Geometry check sheet. Reference: the model listing, model coordinates, mm. A direction names the side the tool comes from. Coordinates: 2 decimals unless noted, no trailing zeros. Write each loop counter-clockwise with the first axis right and the second up, starting at its lowest first coordinate (ties: lowest second). Pieces come first, ordered by that corner, then holes.
from build123d import *

# Parameters (mm, degrees)
SKETCH_W        = 100.5
SKETCH_H        = 50
SKETCH_R        = 1.7
SKETCH_W_2      = 30
SKETCH_H_2      = 40
SKETCH_W_3      = 13
PAD_DEPTH       = 8
SKETCH001_W     = 86.5
SKETCH001_H     = 44
POCKET_DEPTH    = 3
SKETCH002_W     = 96.5
SKETCH002_H     = 2
POCKET001_DEPTH = 4
POCKET003_DEPTH = 5
SKETCH005_R     = 1.7
POCKET004_DEPTH = 3.001
POCKET005_DEPTH = 3
FILLET_R        = 3
FILLET001_R     = 3
FILLET002_R     = 3
FILLET003_R     = 3
SKETCH007_W     = 4
SKETCH007_H     = 35
POCKET006_DEPTH = 3
SKETCH008_R     = 2
POCKET007_DEPTH = 5.001
CHAMFER_SIZE    = 1.5
CHAMFER001_SIZE = 1.5
CHAMFER002_SIZE = 1.5
CHAMFER003_SIZE = 1.5


with BuildPart() as part:
    # Sketch → Pad (new body)
    with BuildSketch(Plane.XY):
        Rectangle(SKETCH_W, SKETCH_H)
        with Locations((-6, 0)):
            Circle(SKETCH_R, mode=Mode.SUBTRACT)
        with Locations((19, 0)):
            Circle(SKETCH_R, mode=Mode.SUBTRACT)
        with Locations((-28.25, 0)):
            Rectangle(SKETCH_W_2, SKETCH_H_2, mode=Mode.SUBTRACT)
        with Locations((36.75, 0)):
            Rectangle(SKETCH_W_3, SKETCH_H_2, mode=Mode.SUBTRACT)
    extrude(amount=PAD_DEPTH)

    # Sketch001 → Pocket (cut)
    with BuildSketch(Plane.XY.offset(8)):
        Rectangle(SKETCH001_W, SKETCH001_H)
    extrude(amount=-POCKET_DEPTH, mode=Mode.SUBTRACT)

    # Sketch002 → Pocket001 (cut)
    with BuildSketch(Plane.XY.offset(8)):
        with Locations((0, 10.5)):
            Rectangle(SKETCH002_W, SKETCH002_H)
        with Locations((0, -4.5)):
            Rectangle(SKETCH002_W, SKETCH002_H)
    extrude(amount=-POCKET001_DEPTH, mode=Mode.SUBTRACT)

    # Sketch004 → Pocket003 (cut)
    with BuildSketch(Plane.XY.offset(8)):
        Polygon((-50.25, 25), (50.25, 25), (50.25, 17), (43.25, 17), (43.25, 22), (-43.25, 22), (-43.25, 17), (-50.25, 17), align=None)
        Polygon((50.25, -17), (50.25, -25), (-50.25, -25), (-50.25, -17), (-43.25, -17), (-43.25, -22), (43.25, -22), (43.25, -17), align=None)
    extrude(amount=-POCKET003_DEPTH, mode=Mode.SUBTRACT)

    # Sketch005 → Pocket004 (cut, through all)
    with BuildSketch(Plane.XY.offset(3)):
        with Locations((-47, 21)):
            Circle(SKETCH005_R)
        with Locations((47, 21)):
            Circle(SKETCH005_R)
        with Locations((47, -21)):
            Circle(SKETCH005_R)
        with Locations((-47, -21)):
            Circle(SKETCH005_R)
    extrude(amount=-POCKET004_DEPTH, mode=Mode.SUBTRACT)

    # Sketch006 → Pocket005 (cut)
    with BuildSketch(Plane.XY.offset(5)):
        Polygon((-7.587713, 2.75), (-9.175426, 0), (-7.587713, -2.75), (-4.412287, -2.75), (-2.824574, 0), (-4.412287, 2.75), align=None)
        Polygon((17.412287, 2.75), (15.824574, 0), (17.412287, -2.75), (20.587713, -2.75), (22.175426, 0), (20.587713, 2.75), align=None)
    extrude(amount=-POCKET005_DEPTH, mode=Mode.SUBTRACT)

    # Fillet
    fillet_edges = [part.edges().sort_by_distance(p)[0] for p in [
        (-50.25, -25, 1.5),
    ]]
    fillet(fillet_edges, radius=FILLET_R)

    # Fillet001
    fillet001_edges = [part.edges().sort_by_distance(p)[0] for p in [
        (-50.25, 25, 1.5),
    ]]
    fillet(fillet001_edges, radius=FILLET001_R)

    # Fillet002
    fillet002_edges = [part.edges().sort_by_distance(p)[0] for p in [
        (50.25, -25, 1.5),
    ]]
    fillet(fillet002_edges, radius=FILLET002_R)

    # Fillet003
    fillet003_edges = [part.edges().sort_by_distance(p)[0] for p in [
        (50.25, 25, 1.5),
    ]]
    fillet(fillet003_edges, radius=FILLET003_R)

    # Sketch007 → Pocket006 (cut)
    with BuildSketch(Plane.XY.offset(5)):
        with Locations((2, 0)):
            Rectangle(SKETCH007_W, SKETCH007_H)
    extrude(amount=-POCKET006_DEPTH, mode=Mode.SUBTRACT)

    # Sketch008 → Pocket007 (cut, through all)
    with BuildSketch(Plane.XY.offset(5)):
        with Locations((2, 17.5)):
            Circle(SKETCH008_R)
        with Locations((2, 0)):
            Circle(SKETCH008_R)
        with Locations((2, -17.5)):
            Circle(SKETCH008_R)
    extrude(amount=-POCKET007_DEPTH, mode=Mode.SUBTRACT)

    # Chamfer
    chamfer_edges = [part.edges().sort_by_distance(p)[0] for p in [
        (-48.7, 21, 0),
    ]]
    chamfer(chamfer_edges, length=CHAMFER_SIZE)

    # Chamfer001
    chamfer001_edges = [part.edges().sort_by_distance(p)[0] for p in [
        (-48.7, -21, 0),
    ]]
    chamfer(chamfer001_edges, length=CHAMFER001_SIZE)

    # Chamfer002
    chamfer002_edges = [part.edges().sort_by_distance(p)[0] for p in [
        (45.3, 21, 0),
    ]]
    chamfer(chamfer002_edges, length=CHAMFER002_SIZE)

    # Chamfer003
    chamfer003_edges = [part.edges().sort_by_distance(p)[0] for p in [
        (45.3, -21, 0),
    ]]
    chamfer(chamfer003_edges, length=CHAMFER003_SIZE)


solid = part.part
1. Access from +Z, -Z, +X, -X, +Y, -Y to the whole of each face (thin tool, end or side, straight path). Record for faces 1 (the flat face through (19, 2.75, 4)), 2 (the cylindrical face through (2.923, -19.274, 1.979)), 3 (the flat face through (-43.25, -21, 4)), 4 (the flat face through (47, 17, 6)).
Computed values:
face 1: +Z
face 2: +Z, -Z
face 3: +Z, -X, -Y
face 4: +Z, +X, +Y
2. Sectioned sample at A-A, the plane x = -33.5. Record the boundary of the cut face in (y, z), and give its area (3 significant figures).
Computed values:
outline: (-25, 0) - (-20, 0) - (-20, 5) - (-22, 5) - (-22, 3) - (-25, 3) - close; (20, 0) - (25, 0) - (25, 3) - (22, 3) - (22, 5) - (20, 5) - close
area: 38.0 mm2
3. Draft check along Y on faces 5 (the flat face through (47, -17, 6)), 6 (the flat face through (-1, 0, 0)), 7 (the flat face through (46, -5.5, 6)). Enter one of: released by +Y, released by -Y, zero draft, split by the parting line, or undercut.
Computed values:
face 5: released by -Y
face 6: zero draft
face 7: undercut
4. Sectioned sample at B-B, the plane y = -9.5. Record the boundary of the cut face in (x, z).
Computed values:
outline: (-50.25, 0) - (-43.25, 0) - (-43.25, 8) - (-50.25, 8) - close; (-13.25, 0) - (30.25, 0) - (30.25, 5) - (4, 5) - (4, 2) - (0, 2) - (0, 5) - (-13.25, 5) - close; (43.25, 0) - (50.25, 0) - (50.25, 8) - (43.25, 8) - close
5. Sectioned sample at C-C, the plane x = 11. Record the boundary of the cut face in (y, z).
Computed values:
outline: (-25, 0) - (25, 0) - (25, 3) - (22, 3) - (22, 5) - (11.5, 5) - (11.5, 4) - (9.5, 4) - (9.5, 5) - (-3.5, 5) - (-3.5, 4) - (-5.5, 4) - (-5.5, 5) - (-22, 5) - (-22, 3) - (-25, 3) - close
6. Gauge pin test, flat ends, axial feed: pin 1 Ø2 at (x, y) = (25, -18) entering from +Z; pin 2 Ø4.5 at (x, y) = (47, -21) entering from +Z; pin 3 Ø0.8 at (x, z) = (10.5, 4.5) entering from -Y. Record the tip position at first contact, or that the pin passes through.
Computed values:
pin 1: stops at z = 5
pin 2: stops at z = 3
pin 3: stops at y = -22
7. Sectioned sample at D-D, the plane y = -21. Record the boundary of the cut face in (x, z).
Computed values:
outline: (-50.25, 0) - (-50.2, 0) - (-48.7, 1.5) - (-48.7, 3) - (-50.25, 3) - close; (-45.3, 1.5) - (-43.8, 0) - (43.8, 0) - (45.3, 1.5) - (45.3, 3) - (43.25, 3) - (43.25, 5) - (-43.25, 5) - (-43.25, 3) - (-45.3, 3) - close; (48.7, 1.5) - (50.2, 0) - (50.25, 0) - (50.25, 3) - (48.7, 3) - close
8. Thickness scan on line 1 along Y through (x, z) = (-47, 2); line 2 along X through (y, z) = (0, 1.55); line 3 along X through (y, z) = (-15.5, 4.5). Record the ranges inside material, lowest first.
Computed values:
line 1: y = -25 to -22.7, -19.3 to 19.3, 22.7 to 25
line 2: x = -50.25 to -43.25, -13.25 to -7.7, -4.3 to 0, 4 to 17.3, 20.7 to 30.25, 43.25 to 50.25
line 3: x = -50.25 to -43.25, -13.25 to 0, 4 to 30.25, 43.25 to 50.25
